```python
from build123d import *

# Parameters (mm, degrees)
EXTRUDE_1_DEPTH     = 10
SKETCH_4_W          = 15
SKETCH_4_H          = 30
CUT_EXTRUDE_2_DEPTH = 5
FILLET_1_R          = 3
CUT_EXTRUDE_3_DEPTH = 111.616454472
HOLE_WIZARD_M41_D   = 4.5
M4X0_72_D           = 3.3


with BuildPart() as part:
    # Эскиз1 → Бобышка-Вытянуть1 (new body)
    with BuildSketch(Plane(origin=(0, 0, 0), x_dir=(1, 0, 0), z_dir=(0, 1, 0))):
        Polygon((15, 0), (106, 0), (106, 30), (15, 30), (10, 30), (0, 29.125113365), (0, 0.874886635), (10, 0), align=None)
    extrude(amount=EXTRUDE_1_DEPTH)

    # Эскиз4 → Вырез-Вытянуть2 (cut)
    with BuildSketch(Plane.XZ):
        with Locations((7.5, -15)):
            Rectangle(SKETCH_4_W, SKETCH_4_H)
    extrude(amount=-CUT_EXTRUDE_2_DEPTH, mode=Mode.SUBTRACT)

    # Скругление1
    # the kernel refuses this fillet: 3 mm, written as the material it takes off along each edge
    with BuildSketch(Plane(origin=(10, 4.672542928, 0), x_dir=(1, 0, 0), z_dir=(0, 1, 0))) as fillet_1_piece_1:
        with BuildLine():
            CenterArc((FILLET_1_R * 0.0436609429085, FILLET_1_R), FILLET_1_R, 265, 5)
            Line((-FILLET_1_R * 0.0434947998391, FILLET_1_R * 0.00380530190825), (0, 0))
            Line((0, 0), (FILLET_1_R * 0.0436609429085, 0))
        make_face()
    extrude(amount=5.654914144, mode=Mode.SUBTRACT)
    with BuildSketch(Plane(origin=(0, -1.872483805, -0.874886635), x_dir=(0.9961946980917452, 0, 0.08715574274766158), z_dir=(0, 1, 0))) as fillet_1_piece_2:
        with BuildLine():
            CenterArc((FILLET_1_R * 0.916331174017, FILLET_1_R), FILLET_1_R, 185, 85)
            Line((-FILLET_1_R * 0.0798635240743, FILLET_1_R * 0.912844257252), (0, 0))
            Line((0, 0), (FILLET_1_R * 0.916331174017, 0))
        make_face()
    extrude(amount=18.74496761, mode=Mode.SUBTRACT)
    with BuildSketch(Plane(origin=(0, -1.872483805, -29.125113365), x_dir=(0.9961946980917452, 0, -0.08715574274766201), z_dir=(0, 1, 0))) as fillet_1_piece_3:
        with BuildLine():
            CenterArc((FILLET_1_R * 0.916331174017, -FILLET_1_R), FILLET_1_R, 90, 85)
            Line((-FILLET_1_R * 0.0798635240743, -FILLET_1_R * 0.912844257252), (0, 0))
            Line((0, 0), (FILLET_1_R * 0.916331174017, 0))
        make_face()
    extrude(amount=18.74496761, mode=Mode.SUBTRACT)
    with BuildSketch(Plane(origin=(10, 4.672542928, -30), x_dir=(1, 0, 0), z_dir=(0, 1, 0))) as fillet_1_piece_4:
        with BuildLine():
            CenterArc((FILLET_1_R * 0.0436609429085, -FILLET_1_R), FILLET_1_R, 90, 5)
            Line((-FILLET_1_R * 0.0434947998391, -FILLET_1_R * 0.00380530190825), (0, 0))
            Line((0, 0), (FILLET_1_R * 0.0436609429085, 0))
        make_face()
    extrude(amount=5.654914144, mode=Mode.SUBTRACT)

    # Эскиз5 → Вырез-Вытянуть3 (cut, through all)
    with BuildSketch(Plane.XZ):
        with BuildLine():
            Line((22.5, -17), (28.5, -17))
            ThreePointArc((28.5, -17), (29.914213562, -17.585786438), (30.5, -19))
            Line((30.5, -19), (30.5, -25))
            ThreePointArc((30.5, -25), (29.914213562, -26.414213562), (28.5, -27))
            Line((28.5, -27), (22.5, -27))
            ThreePointArc((22.5, -27), (21.085786438, -26.414213562), (20.5, -25))
            Line((20.5, -25), (20.5, -19))
            ThreePointArc((20.5, -19), (21.085786438, -17.585786438), (22.5, -17))
        make_face()
        with BuildLine():
            Line((34.5, -17), (40.5, -17))
            ThreePointArc((40.5, -17), (41.914213562, -17.585786438), (42.5, -19))
            Line((42.5, -19), (42.5, -25))
            ThreePointArc((42.5, -25), (41.914213562, -26.414213562), (40.5, -27))
            Line((40.5, -27), (34.5, -27))
            ThreePointArc((34.5, -27), (33.085786438, -26.414213562), (32.5, -25))
            Line((32.5, -25), (32.5, -19))
            ThreePointArc((32.5, -19), (33.085786438, -17.585786438), (34.5, -17))
        make_face()
        with BuildLine():
            Line((46.5, -17), (52.5, -17))
            ThreePointArc((52.5, -17), (53.914213562, -17.585786438), (54.5, -19))
            Line((54.5, -19), (54.5, -25))
            ThreePointArc((54.5, -25), (53.914213562, -26.414213562), (52.5, -27))
            Line((52.5, -27), (46.5, -27))
            ThreePointArc((46.5, -27), (45.085786438, -26.414213562), (44.5, -25))
            Line((44.5, -25), (44.5, -19))
            ThreePointArc((44.5, -19), (45.085786438, -17.585786438), (46.5, -17))
        make_face()
        with BuildLine():
            Line((58.5, -17), (64.5, -17))
            ThreePointArc((64.5, -17), (65.914213562, -17.585786438), (66.5, -19))
            Line((66.5, -19), (66.5, -25))
            ThreePointArc((66.5, -25), (65.914213562, -26.414213562), (64.5, -27))
            Line((64.5, -27), (58.5, -27))
            ThreePointArc((58.5, -27), (57.085786438, -26.414213562), (56.5, -25))
            Line((56.5, -25), (56.5, -19))
            ThreePointArc((56.5, -19), (57.085786438, -17.585786438), (58.5, -17))
        make_face()
        with BuildLine():
            Line((70.5, -17), (76.5, -17))
            ThreePointArc((76.5, -17), (77.914213562, -17.585786438), (78.5, -19))
            Line((78.5, -19), (78.5, -25))
            ThreePointArc((78.5, -25), (77.914213562, -26.414213562), (76.5, -27))
            Line((76.5, -27), (70.5, -27))
            ThreePointArc((70.5, -27), (69.085786438, -26.414213562), (68.5, -25))
            Line((68.5, -25), (68.5, -19))
            ThreePointArc((68.5, -19), (69.085786438, -17.585786438), (70.5, -17))
        make_face()
        with BuildLine():
            Line((82.5, -17), (88.5, -17))
            ThreePointArc((88.5, -17), (89.914213562, -17.585786438), (90.5, -19))
            Line((90.5, -19), (90.5, -25))
            ThreePointArc((90.5, -25), (89.914213562, -26.414213562), (88.5, -27))
            Line((88.5, -27), (82.5, -27))
            ThreePointArc((82.5, -27), (81.085786438, -26.414213562), (80.5, -25))
            Line((80.5, -25), (80.5, -19))
            ThreePointArc((80.5, -19), (81.085786438, -17.585786438), (82.5, -17))
        make_face()
        with BuildLine():
            Line((90.5, -11), (90.5, -5))
            ThreePointArc((90.5, -5), (89.914213562, -3.585786438), (88.5, -3))
            Line((88.5, -3), (82.5, -3))
            ThreePointArc((82.5, -3), (81.085786438, -3.585786438), (80.5, -5))
            Line((80.5, -5), (80.5, -11))
            ThreePointArc((80.5, -11), (81.085786438, -12.414213562), (82.5, -13))
            Line((82.5, -13), (88.5, -13))
            ThreePointArc((88.5, -13), (89.914213562, -12.414213562), (90.5, -11))
        make_face()
        with BuildLine():
            Line((78.5, -11), (78.5, -5))
            ThreePointArc((78.5, -5), (77.914213562, -3.585786438), (76.5, -3))
            Line((76.5, -3), (70.5, -3))
            ThreePointArc((70.5, -3), (69.085786438, -3.585786438), (68.5, -5))
            Line((68.5, -5), (68.5, -11))
            ThreePointArc((68.5, -11), (69.085786438, -12.414213562), (70.5, -13))
            Line((70.5, -13), (76.5, -13))
            ThreePointArc((76.5, -13), (77.914213562, -12.414213562), (78.5, -11))
        make_face()
        with BuildLine():
            Line((66.5, -11), (66.5, -5))
            ThreePointArc((66.5, -5), (65.914213562, -3.585786438), (64.5, -3))
            Line((64.5, -3), (58.5, -3))
            ThreePointArc((58.5, -3), (57.085786438, -3.585786438), (56.5, -5))
            Line((56.5, -5), (56.5, -11))
            ThreePointArc((56.5, -11), (57.085786438, -12.414213562), (58.5, -13))
            Line((58.5, -13), (64.5, -13))
            ThreePointArc((64.5, -13), (65.914213562, -12.414213562), (66.5, -11))
        make_face()
        with BuildLine():
            Line((54.5, -11), (54.5, -5))
            ThreePointArc((54.5, -5), (53.914213562, -3.585786438), (52.5, -3))
            Line((52.5, -3), (46.5, -3))
            ThreePointArc((46.5, -3), (45.085786438, -3.585786438), (44.5, -5))
            Line((44.5, -5), (44.5, -11))
            ThreePointArc((44.5, -11), (45.085786438, -12.414213562), (46.5, -13))
            Line((46.5, -13), (52.5, -13))
            ThreePointArc((52.5, -13), (53.914213562, -12.414213562), (54.5, -11))
        make_face()
        with BuildLine():
            Line((42.5, -11), (42.5, -5))
            ThreePointArc((42.5, -5), (41.914213562, -3.585786438), (40.5, -3))
            Line((40.5, -3), (34.5, -3))
            ThreePointArc((34.5, -3), (33.085786438, -3.585786438), (32.5, -5))
            Line((32.5, -5), (32.5, -11))
            ThreePointArc((32.5, -11), (33.085786438, -12.414213562), (34.5, -13))
            Line((34.5, -13), (40.5, -13))
            ThreePointArc((40.5, -13), (41.914213562, -12.414213562), (42.5, -11))
        make_face()
        with BuildLine():
            Line((30.5, -11), (30.5, -5))
            ThreePointArc((30.5, -5), (29.914213562, -3.585786438), (28.5, -3))
            Line((28.5, -3), (22.5, -3))
            ThreePointArc((22.5, -3), (21.085786438, -3.585786438), (20.5, -5))
            Line((20.5, -5), (20.5, -11))
            ThreePointArc((20.5, -11), (21.085786438, -12.414213562), (22.5, -13))
            Line((22.5, -13), (28.5, -13))
            ThreePointArc((28.5, -13), (29.914213562, -12.414213562), (30.5, -11))
        make_face()
    extrude(amount=-CUT_EXTRUDE_3_DEPTH, mode=Mode.SUBTRACT)

    # Отверстие с зазором M41 (through all)
    with Locations(Plane(origin=(0, 10, 0), x_dir=(1, 0, 0), z_dir=(0, 1, 0))):
        with Locations((101, 25), (101, 5)):
            Hole(HOLE_WIZARD_M41_D / 2)

    # Отверстие обработанное метчиком M4x0.72 (through all)
    with Locations(Plane(origin=(0, 10, 0), x_dir=(1, 0, 0), z_dir=(0, 1, 0))):
        with Locations((7.5, 22.390639171), (7.5, 7.609360829)):
            Hole(M4X0_72_D / 2)


solid = part.part
```
The listing builds one solid part. Answer for the finished solid, in the listing's coordinates (mm). Round coordinates to 2 decimals unless told otherwise and drop trailing zeros. Write each loop counter-clockwise with the first axis right and the second up, starting at its lowest first coordinate (ties: lowest second). Pieces come first, ordered by that corner, then holes. Notation, with made-up numbers: (50, 73.5) -> (58, 73.5) arc R22 cw to (58, 82.5) -> close; hole circle Ø5 at (65, -33). An arc over 180 degrees is marked (long way). Answer as a JSON object with one key per item and string values. Group by question number.
Q1. Section A-A (x = 101) is taken. Write down the section's boundary in (y, z).
Q2. Section C-C (y = 1.75) is taken. Count the separate pieces of the cut face and the enclosed holes in it, plus the area to 3 significant figures.
Q3. Section B-B (z = -15.5) is taken. Write down the section's boundary in (x, y), plus the area to 3 significant figures.
Q4. Determine the mould class of faces 1 (the face through (57.1, 4.93, -26.43)), 2 (the face through (0.77, 7.46, -1.62)) for opening direction Z: pulls with the +Z half, pulls with the -Z half, needs draft (parallel to the pull), parting line crosses it, or undercut.
Q5. Straight lines are drawn through the part: line 1 along Z through (x, y) = (22.5, 0.75); line 2 along Z through (x, y) = (101, 6.25); line 3 along X through (y, z) = (0.75, -13.75). For each, find the intervals that lie inside material, in ascending order.
Q6. Section D-D (x = 7.5) is taken. Write down the section's boundary in (y, z).
Q7. This flat-tipped pin is pushed along its axis until it touches: pin 1 Ø5 at (y, z) = (4.5, -17) entering from -X. Where does it stop, or does it pass through?
Check values:
{
 "1": {"outline": "(0, -30) -> (10, -30) -> (10, -27.25) -> (0, -27.25) -> close; (0, -22.75) -> (10, -22.75) -> (10, -7.25) -> (0, -7.25) -> close; (0, -2.75) -> (10, -2.75) -> (10, 0) -> (0, 0) -> close"},
 "2": {"separate pieces": "1", "enclosed holes": "14", "area": "1,540 mm^2"},
 "3": {"outline": "(0, 5) -> (15, 5) -> (15, 0) -> (106, 0) -> (106, 10) -> (0, 10) -> close", "area": "985 mm^2"},
 "4": {"face 1": "undercut", "face 2": "pulls with the +Z half"},
 "5": {"line 1": "-30 to -27, -17 to -13, -3 to 0", "line 2": "-30 to -27.25, -22.75 to -7.25, -2.75 to 0", "line 3": "15 to 106"},
 "6": {"outline": "(5, -29.78) -> (10, -29.78) -> (10, -24.04) -> (5, -24.04) -> close; (5, -20.74) -> (10, -20.74) -> (10, -9.26) -> (5, -9.26) -> close; (5, -5.96) -> (10, -5.96) -> (10, -0.22) -> (5, -0.22) -> close"},
 "7": {"pin 1": "x = 0"}
}
